Geometry: final body of the model. Coordinates: model frame, mm. A direction names the side the tool comes from. Give positions to 0.01 mm unless a question says otherwise; leave off trailing zeros. Write each loop counter-clockwise with the first axis right and the second up, starting at its lowest first coordinate (ties: lowest second). Pieces come first, ordered by that corner, then holes. Notation, with made-up numbers: M 45.25,-26.75 L 97.25,-26.75 A27 cw 97.25,-5.75 Z; hole C -3,45 d9. An arc over 180 degrees is marked long. Use one line per item in the form item = value. Start each with the question number.
Item 1: Pull-direction query (X, two-part tool) for faces 1 (the flat face through (0, 25, 20)), 2 (the flat face through (0, 24.5, 4)), 3 (the flat face through (-30, 9, 2)); classes: released by +X, released by -X, zero draft, split by the parting line, or undercut.
Item 2: Access query for faces 4 (the flat face through (30, 9, 2)), 5 (the cylindrical face through (-0.454, -0.35, 12.864)), 6 (the cylindrical face through (0.414, 0.096, 10.365)). Directions: +Z, -Z, +X, -X, +Y, -Y. A direction counts if a zero-diameter tool reaches every point of the face in a straight line with its end or side. Return the directions, or none.
Item 3: Section query C-C on y = -14.5. Return loops of the section in (x, z).
Item 4: Contact query for flat-ended pins moving along their axis: P1, Ø6, axis at x = 11.5, y = 11.5, coming from the -Z side; P2, Ø12, axis at x = 7, z = 25, coming from the -Y side; P3, Ø12, axis at x = -14.5, y = 0.5, coming from the -Z side. Output: stop coordinate, or through.
Item 5: Section query B-B on z = 26.5. Return loops of the section in (x, y), then the cut area to 3 significant figures.
Item 6: Section query D-D on x = -23. Return loops of the section in (y, z).
Item 7: Section query A-A on x = 0. Return loops of the section in (y, z).
Item 8: Material intervals for line 1 along Z through (x, y) = (0, 25.5); line 2 along Y through (x, z) = (-4, 15); line 3 along Z through (x, y) = (-1, 0), sorted ascending. Write a range as from..to.
from build123d import *

# Parameters (mm, degrees)
F0_W     = 60
F0_H     = 50
F1_DEPTH = 25
F3_DEPTH = 50.001
F4_W     = 60
F4_H     = 30.659744516
F5_DEPTH = 2
F6_R     = 2
F7_DEPTH = 2.001
F8_T     = -2.5
F9_DEPTH = 25


# Not quite as in the source:
# - a feature of the source that left no trace in its solid (it failed there, or was rolled back) is left out


with BuildPart() as f1:
    # F0 (on Top) → F1 (new body)
    with BuildSketch(Plane.XY):
        Rectangle(F0_W, F0_H)
    extrude(amount=F1_DEPTH)

    # F2 (on face) → F3 (cut, through all)
    with BuildSketch(Plane.XZ.offset(25)):
        with BuildLine():
            ThreePointArc((-30, 2.2523000371), (0, 12.8664154965), (30, 2.2523000371))
            Line((30, 2.2523000371), (30, 25))
            Line((30, 25), (-30, 25))
            Line((-30, 25), (-30, 2.2523000371))
        make_face()
    extrude(amount=-F3_DEPTH, mode=Mode.SUBTRACT)

    # F4 (on face) → F5 (join)
    with BuildSketch(Plane(origin=(0, 25, 0), x_dir=(-1, 0, 0), z_dir=(0, 1, 0))):
        with Locations((0, 15.329872258)):
            Rectangle(F4_W, F4_H)
    extrude(amount=F5_DEPTH)

    # F6 (on face) → F7 (cut, through all)
    with BuildSketch(Plane.XZ.offset(-25)):
        with Locations((0, 25.7051046938)):
            Circle(F6_R)
    extrude(amount=-F7_DEPTH, mode=Mode.SUBTRACT)

    # F8
    f8_openings = [f1.faces().sort_by_distance(p)[0] for p in [
        (0, 1, 0),
    ]]
    offset(amount=F8_T, openings=f8_openings)

    # F9 (cut): a face of the model
    f9_faces = [f1.faces().sort_by_distance(p)[0] for p in [
        (0, -22.5, 4.2031942767),
    ]]
    extrude(f9_faces, amount=-F9_DEPTH, mode=Mode.SUBTRACT)


solid = f1.part
Answer sheet:
q1.face_1 = zero draft
q1.face_2 = undercut
q1.face_3 = released by -X
q2.face_4 = +Z, -Z, +X, +Y, -Y
q2.face_5 = +Z, -Y
q2.face_6 = -Z, -Y
q3.outline = M -30,0 L -27.5,0 L -27.5,1.04 A45.2 cw 27.5,1.04 L 27.5,0 L 30,0 L 30,2.25 A47.7 ccw -30,2.25 Z
q4.P1 = 7.98
q4.P2 = 25
q4.P3 = 5.45
q5.outline = M -30,25 L -1.84,25 L -1.84,27 L -30,27 Z; M 1.84,25 L 30,25 L 30,27 L 1.84,27 Z
q5.area = 113 mm2
q6.outline = M -25,4.08 L 24.5,4.08 L 24.5,0 L 27,0 L 27,30.66 L 25,30.66 L 25,6.96 L -25,6.96 Z
q7.outline = M -25,10.37 L 24.5,10.37 L 24.5,0 L 27,0 L 27,23.71 L 25,23.71 L 25,12.87 L -25,12.87 Z; M 25,27.71 L 27,27.71 L 27,30.66 L 25,30.66 Z
q8.line_1 = 0..23.71, 27.71..30.66
q8.line_2 = 25..27
q8.line_3 = 10.36..12.86
